Read the model definition and answer for the solid it produces. Units are mm, in the model's axes. A direction names the side the tool comes from. Give positions to 0.01 mm unless a question says otherwise; leave off trailing zeros. Write each loop counter-clockwise with the first axis right and the second up, starting at its lowest first coordinate (ties: lowest second). Pieces come first, ordered by that corner, then holes. Notation, with made-up numbers: M 39.5,-33.5 L 79.5,-33.5 A18 ccw 79.5,-11.5 Z; hole C -4.75,-1 d4. An arc over 180 degrees is marked long. Put each result on its own line as item: value.
from build123d import *

# Parameters (mm, degrees)
SKETCH1_W             = 86
SKETCH1_H             = 70
BOSS_EXTRUDE1_DEPTH   = 1.5
FILLET1_R             = 2
SKETCH2_W             = 20
SKETCH2_H             = 20
BOSS_EXTRUDE2_DEPTH   = 22
F_1_0MM_DOWEL_HOLE1_D = 3


with BuildPart() as part:
    # Sketch1 → Boss-Extrude1 (new body)
    with BuildSketch(Plane(origin=(0, 0, 0), x_dir=(1, 0, 0), z_dir=(0, 1, 0))):
        Rectangle(SKETCH1_W, SKETCH1_H)
    extrude(amount=BOSS_EXTRUDE1_DEPTH)

    # Fillet1
    fillet1_edges = [part.edges().sort_by_distance(p)[0] for p in [
        (43, 0.75, 35),
        (-43, 0.75, 35),
        (-43, 0.75, -35),
        (43, 0.75, -35),
    ]]
    fillet(fillet1_edges, radius=FILLET1_R)

    # Sketch2 → Boss-Extrude2 (add)
    with BuildSketch(Plane.XZ):
        Rectangle(SKETCH2_W, SKETCH2_H)
    extrude(amount=-BOSS_EXTRUDE2_DEPTH)

    # Ø1.0mm Dowel Hole1 (through all)
    with Locations(Plane(origin=(-39.4, 1.5, -31.4), x_dir=(0, 0, 1), z_dir=(0, 1, 0))):
        with Locations((0, 0), (0, 78.8), (62.8, 0), (62.8, 78.8)):
            Hole(F_1_0MM_DOWEL_HOLE1_D / 2)


solid = part.part
(1) Section D-D on x = 25.5 is taken. Determine the outline of the cut face in (y, z), and give its area (3 significant figures).
Result:
outline: M 0,-35 L 1.5,-35 L 1.5,35 L 0,35 Z
area: 105 mm²
(2) Straight lines are drawn through the part: line 1 along X through (y, z) = (0.7, 31.4); line 2 along Y through (x, z) = (-21, 0); line 3 along X through (y, z) = (10, -8). For each, find the intervals that lie inside material, in ascending order. Write a range as from..to.
Result:
line 1: x = -43..-40.9, -37.9..37.9, 40.9..43
line 2: y = 0..1.5
line 3: x = -10..10
(3) Given pin 1 Ø6 at (y, z) = (15, -3.5) entering from -X; pin 2 Ø12 at (y, z) = (9, -24.5) entering from -X; pin 3 Ø10 at (x, y) = (5, 14.5) entering from -Z; pin 4 Ø1 at (y, z) = (7, 5.5) entering from +X, each flat-ended and moving along its own axis, determine where each tip first touches the part or whether it passes through.
Result:
pin 1: stops at x = -10
pin 2: passes through
pin 3: stops at z = -10
pin 4: stops at x = 10
(4) Section B-B on z = -31.4 is taken. Determine the outline of the cut face in (x, y), and give its area (3 significant figures).
Result:
outline: M -43,0 L -40.9,0 L -40.9,1.5 L -43,1.5 Z; M -37.9,0 L 37.9,0 L 37.9,1.5 L -37.9,1.5 Z; M 40.9,0 L 43,0 L 43,1.5 L 40.9,1.5 Z
area: 120 mm²
(5) For a pull along Z with two mould halves and no side action, classify faces 1 (the face through (-39.33, 0.74, 32.9)), 2 (the face through (-1, 0, 0)), 3 (the face through (42.43, 0.76, -34.4)) as +Z half, -Z half, draft (parallel to the pull), parting line (faces both ways), or undercut.
Result:
face 1: undercut
face 2: draft
face 3: -Z half
(6) Section A-A on x = -39.4 is taken. Determine the outline of the cut face in (y, z), and give its area (3 significant figures).
Result:
outline: M 0,-35 L 1.5,-35 L 1.5,-32.9 L 0,-32.9 Z; M 0,-29.9 L 1.5,-29.9 L 1.5,29.9 L 0,29.9 Z; M 0,32.9 L 1.5,32.9 L 1.5,35 L 0,35 Z
area: 96.0 mm²
(7) Section C-C on z = -8.5 is taken. Determine the outline of the cut face in (x, y).
Result:
outline: M -43,0 L 43,0 L 43,1.5 L 10,1.5 L 10,22 L -10,22 L -10,1.5 L -43,1.5 Z
(8) Which of the six approach directions +Z, -Z, +X, -X, +Y, -Y give full straight-line access (tool end or side, diameter ignored) to faces 4 (the face through (0, 12, 10)), 5 (the face through (-10, 12, 0)), 6 (the face through (0, 12, -10)), 7 (the face through (10, 12, 0))?
Result:
face 4: +Z, +X, -X, +Y
face 5: +Z, -Z, -X, +Y
face 6: -Z, +X, -X, +Y
face 7: +Z, -Z, +X, +Y
